Verification items for the finished model (mm, model axes). A direction names the side the tool comes from. Give positions to 0.01 mm unless a question says otherwise; leave off trailing zeros. Loops run counter-clockwise (first coordinate to the right, second up) from the corner with the lowest first, then second, coordinate; pieces in that order, holes last. Notation, with made-up numbers: M 72.5,63 L 90.5,63 A23 ccw 90.5,96 Z; hole C 55.25,-12.75 d11. An arc over 180 degrees is marked long. Answer in a Markdown table with one row per item.
Autodesk Inventor part; units mm, degrees
ref_plane "YZ Plane" through (0, 0, 0) normal (1, 0, 0) x (0, 1, 0)
ref_plane "XZ Plane" through (0, 0, 0) normal (0, 1, 0) x (-1, 0, 0)
ref_plane "XY Plane" through (0, 0, 0) normal (0, 0, 1) x (1, 0, 0)
sketch "Sketch1" plane through (0, 0, 0) normal (0, 1, 0) x (-1, 0, 0)
  line L0 (232.1908, -176.5808) -> (232.1908, -3.7592)
  arc A0 (232.1908, -3.7592) -> (227.4316, 1) centre (227.4316, -3.7592) ccw
  line L1 (227.4316, 1) -> (0, 1)
  arc A1 (0, 1) -> (-4.7592, -3.7592) centre (0, -3.7592) ccw
  arc A2 (-4.7592, -176.5808) -> (0, -181.34) centre (0, -176.5808) ccw
  arc A3 (227.4316, -181.34) -> (232.1908, -176.5808) centre (227.4316, -176.5808) ccw
  circle A4 centre (130, -129.34) radius 2.25
  circle A5 centre (129.9861, -89.34) radius 2.25
  circle A6 centre (90, -129.34) radius 2.25
  circle A7 centre (89.9861, -89.34) radius 2.25
  circle A8 centre (180, -110) radius 2.75
  circle A9 centre (55, -110) radius 2.75
  circle A10 centre (90, -45) radius 3
  circle A11 centre (190, -45) radius 3
  circle A12 centre (190, -65) radius 3
  circle A13 centre (90, -65) radius 3
  circle A14 centre (140, -45) radius 3
  circle A15 centre (40, -45) radius 3
  circle A16 centre (140, -65) radius 3
  circle A17 centre (40, -65) radius 3
  line L2 (230.1908, -176.5808) -> (230.1908, -3.7592)
  arc A18 (230.1908, -3.7592) -> (227.4316, -1) centre (227.4316, -3.7592) ccw
  line L3 (227.4316, -1) -> (0, -1)
  arc A19 (0, -1) -> (-2.7592, -3.7592) centre (0, -3.7592) ccw
  arc A20 (-2.7592, -176.5808) -> (0, -179.34) centre (0, -176.5808) ccw
  arc A21 (227.4316, -179.34) -> (230.1908, -176.5808) centre (227.4316, -176.5808) ccw
  line L4 (-4.7592, -3.7592) -> (-4.7592, -176.5808)
  line L5 (-2.7592, -3.7592) -> (-2.7592, -176.5808)
  line L6 (0, -179.34) -> (227.4316, -179.34)
  line L7 (227.4316, -181.34) -> (0, -181.34)
  line L8 (0, 0) -> (0, -15)
  line L9 (0, 0) -> (15, 0) construction
  line L10 (0, 0) -> (15, 0)
  line L11 (0, 0) -> (15, 0) construction
  circle A22 centre (20, -155) radius 2.25
  circle A23 centre (76, -155) radius 2.25
  circle A24 centre (20, -99) radius 2.25
  point P0 (230.1908, -3.7592)
  point P1 (0, -1)
  dimension "d0" = 2
  dimension "d1" = 2
  dimension "d2" = 2
  dimension "d3" = 2
  dimension "d5" = 2
  dimension "d7" = 2
  dimension "d8" = 227.4316
  dimension "d9" = 172.8216
  dimension "d10" = 4.7592
  dimension "d45" = 15
  dimension "d46" = 90
  dimension "d47" = 15
  dimension "d48" = 0
  dimension "d49" = 110
  dimension "d50" = 55
  dimension "d51" = 125
  dimension "d52" = 110
  dimension "d54" = 40
  dimension "d55" = 40
  dimension "d56" = 40
  dimension "d57" = 40
  dimension "d58" = 50
  dimension "d59" = 100.1908
  dimension "d60" = 2.7592
  dimension "d61" = 1
  dimension "d62" = 4.7592
  dimension "d63" = 178.34
  dimension "d64" = 180.34
  dimension "d65" = 172.8216
  dimension "d66" = 230.1908
  dimension "d67" = 4.5
  dimension "d68" = 5.5
  dimension "d69" = 6
  dimension "d70" = 40.1908
  dimension "d71" = 64
  dimension "d72" = 20
  dimension "d73" = 50
  dimension "d74" = 50
  dimension "d75" = 50
  dimension "d76" = 20
  dimension "d77" = 20
  dimension "d78" = 20
  dimension "d79" = 50
  dimension "d87" = 4.5
  dimension "d89" = 45
  dimension "d90" = 35
  dimension "d91" = 4.5
  dimension "d92" = 56
  dimension "d93" = 4.5
  dimension "d94" = 56
extrude "Extrusion1" add sketch "Sketch1" along normal blind 6 contours A21 L6 A20 L5 A19 L3 A18 L2
sketch "Sketch2" plane through (0, 6, 0) normal (0, 1, 0) x (1, 0, 0)
  line L0 (-232.1908, 176.5808) -> (-232.1908, 3.7592)
  arc A0 (-232.1908, 3.7592) -> (-227.4316, -1) centre (-227.4316, 3.7592) ccw
  line L1 (-227.4316, -1) -> (0, -1)
  arc A1 (0, -1) -> (4.7592, 3.7592) centre (0, 3.7592) ccw
  arc A2 (4.7592, 176.5808) -> (0, 181.34) centre (0, 176.5808) ccw
  arc A3 (-227.4316, 181.34) -> (-232.1908, 176.5808) centre (-227.4316, 176.5808) ccw
  circle A4 centre (-130, 135) radius 2
  circle A5 centre (-130, 95) radius 2
  circle A6 centre (-90, 135) radius 2
  circle A7 centre (-90, 95) radius 2
  circle A8 centre (-160.0797, 100) radius 2.75
  circle A9 centre (-60.0797, 100) radius 2.75
  circle A10 centre (-90, 45) radius 2.5
  circle A11 centre (-190, 45) radius 2.5
  circle A12 centre (-190, 65) radius 2.5
  circle A13 centre (-90, 65) radius 2.5
  circle A14 centre (-140, 45) radius 2.5
  circle A15 centre (-40, 45) radius 2.5
  circle A16 centre (-140, 65) radius 2.5
  circle A17 centre (-40, 65) radius 2.5
  line L2 (-230.1908, 176.5808) -> (-230.1908, 3.7592)
  arc A18 (-230.1908, 3.7592) -> (-227.4316, 1) centre (-227.4316, 3.7592) ccw
  line L3 (-227.4316, 1) -> (0, 1)
  arc A19 (0, 1) -> (2.7592, 3.7592) centre (0, 3.7592) ccw
  arc A20 (2.7592, 176.5808) -> (0, 179.34) centre (0, 176.5808) ccw
  arc A21 (-227.4316, 179.34) -> (-230.1908, 176.5808) centre (-227.4316, 176.5808) ccw
  line L4 (4.7592, 3.7592) -> (4.7592, 176.5808)
  line L5 (2.7592, 3.7592) -> (2.7592, 176.5808)
  line L6 (0, 179.34) -> (-227.4316, 179.34)
  line L7 (-227.4316, 181.34) -> (0, 181.34)
  line L8 (0, 179.34) -> (-227.4316, 179.34)
  line L9 (-113.7158, 179.34) -> (-113.7158, 1)
  line L10 (-227.4316, 1) -> (0, 1)
  line L11 (-118.7158, 120.17) -> (-108.7158, 120.17)
  line L12 (-108.7158, 120.17) -> (-108.7158, 60.17)
  line L13 (-108.7158, 60.17) -> (-118.7158, 60.17)
  line L14 (-118.7158, 60.17) -> (-118.7158, 120.17)
  line L15 (-118.7158, 120.17) -> (-108.7158, 60.17) construction
  line L16 (-108.7158, 120.17) -> (-118.7158, 60.17) construction
  line L17 (-113.7158, 179.34) -> (-113.7158, 179.34)
  line L18 (2.7592, 159.34) -> (-230.1908, 159.34)
  line L19 (-230.1908, 159.34) -> (-230.1908, 199.34)
  line L20 (-230.1908, 199.34) -> (2.7592, 199.34)
  line L21 (2.7592, 199.34) -> (2.7592, 159.34)
  line L22 (2.7592, 159.34) -> (-230.1908, 199.34) construction
  line L23 (-230.1908, 159.34) -> (2.7592, 199.34) construction
  line L24 (-113.7158, 1) -> (-113.7158, 16)
  line L25 (-230.1908, 31) -> (2.7592, 31)
  line L26 (2.7592, 31) -> (2.7592, 1)
  line L27 (2.7592, 1) -> (-230.1908, 1)
  line L28 (-230.1908, 1) -> (-230.1908, 31)
  line L29 (-230.1908, 31) -> (2.7592, 1) construction
  line L30 (2.7592, 31) -> (-230.1908, 1) construction
  line L31 (-227.4316, 1) -> (0, 1)
  line L32 (-230.1908, 199.34) -> (-200.1908, 199.34)
  line L33 (-200.1908, 199.34) -> (-200.1908, 1)
  line L34 (-200.1908, 1) -> (-230.1908, 1)
  line L35 (-230.1908, 1) -> (-230.1908, 199.34)
  line L36 (2.7592, 1) -> (-7.2408, 1)
  line L37 (-7.2408, 1) -> (-7.2408, 199.34)
  line L38 (-7.2408, 199.34) -> (2.7592, 199.34)
  line L39 (2.7592, 199.34) -> (2.7592, 1)
  point P0 (230.1908, -176.5808)
  point P1 (230.1908, -3.7592)
  point P2 (227.4316, -1)
  point P3 (0, -1)
  point P4 (0, 0)
  point P5 (230.1908, -176.5808)
  point P6 (230.1908, -3.7592)
  point P7 (227.4316, -1)
  point P8 (0, -1)
  point P9 (-113.7158, 90.17)
  point P10 (-113.7158, 120.17)
  point P11 (-113.7158, 60.17)
  point P12 (-113.7158, 1)
  point P13 (0, 1)
  point P14 (-230.1908, 3.7592)
  point P15 (-227.4316, 1)
  point P16 (-113.7158, 159.34)
  point P17 (-7.2408, 159.34)
  point P18 (-7.2408, 31)
  point P19 (-113.7158, 31)
  dimension "d22" = 2
  dimension "d23" = 2
  dimension "d24" = 2
  dimension "d25" = 2
  dimension "d26" = 2
  dimension "d27" = 2
  dimension "d28" = 227.4316
  dimension "d29" = 172.8216
  dimension "d30" = 4.7592
  dimension "d31" = 10
  dimension "d32" = 60
  dimension "d37" = 0
  dimension "d38" = 40
  dimension "d39" = 15
  dimension "d40" = 30
  dimension "d41" = 30
  dimension "d42" = 10
extrude "Extrusion3" cut sketch "Sketch2" against normal through all contours A21 L6 L33 L18 L2 | L18 L33 L25 L2 | L6 L9 L18 L33 | L25 L33 L3 A18 L2 | L18 L9 L11 L14 L13 L25 L33 | L37 L18 L9 L6 | L6 A20 L5 L18 L37 | L25 L9 L3 L33 | L18 L5 L25 L37 | L25 L37 L3 L9 | L25 L5 A19 L3 L37 | A4 | A5 | A8 | A11 | A12 | A14 | A16
fillet "Fillet3" radius 2 6 edges at (-113.7158, 3, -31) (-118.7158, 3, -60.17) (-118.7158, 3, -120.17) (-7.2408, 3, -31) (-7.2408, 3, -159.34) (-113.7158, 3, -159.34)
equation "\"d1\" = d0"
equation "\"d2\" = d0"
equation "\"d3\" = d0"
equation "\"d5\" = d0"
equation "\"d7\" = d0"
equation "\"d23\" = d22"
equation "\"d24\" = d22"
equation "\"d25\" = d22"
equation "\"d26\" = d22"
equation "\"d27\" = d22"
properties part number "EboxBottom_2"
Item 1: Sectioned sample at B-B (x = -76). Record the cut outline in (y, z).
Reported:
| item | result |
|---|---|
| outline | M 0,-159.34 L 6,-159.34 L 6,-157.25 L 0,-157.25 Z; M 0,-152.75 L 6,-152.75 L 6,-31 L 0,-31 Z |
Item 2: Release check for a two-part mould opening along Z. For faces 3 (the cylindrical face through (-77.038, 2.958, -153.004)), 4 (the flat face through (-115, 3, -60.17)), 5 (the flat face through (-115, 3, -120.17)) record: released by +Z, released by -Z, zero draft, split by the parting line, or undercut.
Reported:
| item | result |
|---|---|
| face 3 | undercut |
| face 4 | released by +Z |
| face 5 | released by -Z |
Item 3: Sectioned sample at A-A (z = -129.34). Record the cut outline in (x, y).
Reported:
| item | result |
|---|---|
| outline | M -113.72,0 L -92.25,0 L -92.25,6 L -113.72,6 Z; M -87.75,0 L -7.24,0 L -7.24,6 L -87.75,6 Z |
Item 4: Scan lines: L1, parallel to X at y = 4.8, z = -155; L2, parallel to Z at x = -55, y = 2.05; L3, parallel to Z at x = -90, y = 2.4. Record each from-to range of solid material in increasing order. Write a range as [from, to].
Reported:
| item | result |
|---|---|
| L1 | x = [-113.72, -78.25], [-73.75, -22.25], [-17.75, -7.24] |
| L2 | z = [-159.34, -112.75], [-107.25, -31] |
| L3 | z = [-159.34, -131.59], [-127.09, -91.59], [-87.09, -68], [-62, -48], [-42, -31] |
Item 5: Tool access check on faces 1 (the cylindrical face through (-92.08, 2.96, -128.48)), 2 (the flat face through (-113.716, 3, -47)). Record the directions out of +Z, -Z, +X, -X, +Y, -Y that give a thin tool (end or side, any length) a straight path to the whole face; none if there is none.
Reported:
| item | result |
|---|---|
| face 1 | +Y, -Y |
| face 2 | +Z, -X, +Y, -Y |
Item 6: Go/stop test with flat-tipped pins: pin 1 (9.5 mm diameter, centred on x = -40, z = -45, fed in from -Y); pin 2 (0.9 mm diameter, centred on x = -115.5, y = 4, fed in from -Z); pin 3 (3 mm diameter, centred on y = 3, z = -133.5, fed in from -X); pin 4 (0.9 mm diameter, centred on x = -115, y = 2.5, fed in from +Z). Record where each tip stops, or that it passes through.
Reported:
| item | result |
|---|---|
| pin 1 | stops at y = 0 |
| pin 2 | stops at z = -120.17 |
| pin 3 | stops at x = -113.72 |
| pin 4 | stops at z = -60.17 |
Item 7: Sectioned sample at C-C (z = -45). Record the cut outline in (x, y).
Reported:
| item | result |
|---|---|
| outline | M -113.72,0 L -93,0 L -93,6 L -113.72,6 Z; M -87,0 L -43,0 L -43,6 L -87,6 Z; M -37,0 L -7.24,0 L -7.24,6 L -37,6 Z |
Item 8: Sectioned sample at D-D (y = 4.75). State how many separate pieces and enclosed holes the cut face has, and give its area (3 significant figures).
Reported:
| item | result |
|---|---|
| separate pieces | 1 |
| enclosed holes | 10 |
| area | 13,700 mm^2 |
